Study the drawing (mm; zero at the part's minimum x, y, z) and answer. A direction names the side the tool comes from. Coordinates: 2 decimals unless noted, no trailing zeros. Write each loop counter-clockwise with the first axis right and the second up, starting at its lowest first coordinate (ties: lowest second). Pieces come first, ordered by that corner, then holes. Notation, with made-up numbers: (79, 81.5) -> (125, 81.5) arc R26 ccw to (125, 102.5) -> close; hole circle Ø6 at (-38, 77.25). An arc over 180 degrees is marked (long way). Answer in a Markdown table with one row per item. Add a question column.
Item 1: Given pin 1 Ø1 at (x, y) = (32, 1) entering from +Z; pin 2 Ø0.8 at (y, z) = (1.5, 25.5) entering from -X; pin 3 Ø1 at (x, y) = (10.5, 1) entering from +Z, each flat-ended and moving along its own axis, determine where each tip first touches the part or whether it passes through.
Item 2: For a pull along X with two mould halves and no side action, classify the marked faces 5, 6, 7 and 8 as +X half, -X half, draft (parallel to the pull), parting line (faces both ways), or undercut.
Item 3: Section C-C on z = 31 is taken. Write down the section's boundary in (x, y), then the cut area to 3 significant figures.
Item 4: Section B-B on x = 9.5 is taken. Write down the section's boundary in (y, z), then the cut area to 3 significant figures.
Item 5: Which of the six approach directions +Z, -Z, +X, -X, +Y, -Y give full straight-line access (tool end or side, diameter ignored) to the marked faces 1, 2, 3 and 4?
Item 6: Section A-A on y = 2.6 is taken. Write down the section's boundary in (x, z), then the cut area to 3 significant figures.
Item 7: Straight lines are drawn through the part: line 1 (Z direction, x = 6.5, y = 0.2); line 2 (Z direction, x = 22.5, y = 1.3); line 3 (X direction, y = 0.15, z = 2.5). For each, find the intervals that lie inside material, in ascending order. Write a range as from..to.
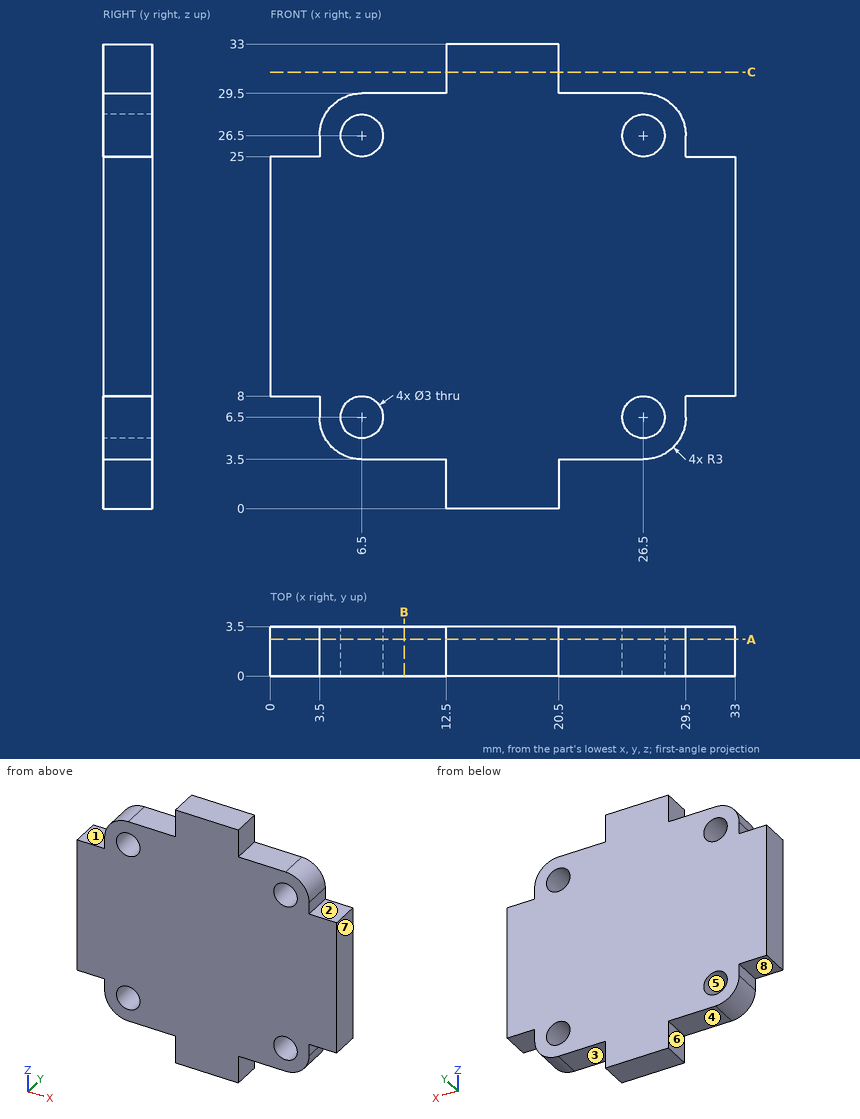
Results below:
| question | item | result |
|---|---|---|
| 1 | pin 1 | stops at z = 25 |
| 1 | pin 2 | stops at x = 3.5 |
| 1 | pin 3 | stops at z = 29.5 |
| 2 | face 5 | undercut |
| 2 | face 6 | -X half |
| 2 | face 7 | +X half |
| 2 | face 8 | draft |
| 3 | outline | (12.5, 0) -> (20.5, 0) -> (20.5, 3.5) -> (12.5, 3.5) -> close |
| 3 | area | 28.0 mm2 |
| 4 | outline | (0, 3.5) -> (3.5, 3.5) -> (3.5, 29.5) -> (0, 29.5) -> close |
| 4 | area | 91.0 mm2 |
| 5 | face 1 | +Z, -X, +Y, -Y |
| 5 | face 2 | +Z, +X, +Y, -Y |
| 5 | face 3 | -Z, +X, +Y, -Y |
| 5 | face 4 | -Z, -X, +Y, -Y |
| 6 | outline | (0, 8) -> (3.5, 8) -> (3.5, 6.5) arc R3 ccw to (6.5, 3.5) -> (12.5, 3.5) -> (12.5, 0) -> (20.5, 0) -> (20.5, 3.5) -> (26.5, 3.5) arc R3 ccw to (29.5, 6.5) -> (29.5, 8) -> (33, 8) -> (33, 25) -> (29.5, 25) -> (29.5, 26.5) arc R3 ccw to (26.5, 29.5) -> (20.5, 29.5) -> (20.5, 33) -> (12.5, 33) -> (12.5, 29.5) -> (6.5, 29.5) arc R3 ccw to (3.5, 26.5) -> (3.5, 25) -> (0, 25) -> close; hole circle Ø3 at (6.5, 6.5); hole circle Ø3 at (6.5, 26.5); hole circle Ø3 at (26.5, 6.5); hole circle Ø3 at (26.5, 26.5) |
| 6 | area | 815 mm2 |
| 7 | line 1 | z = 3.5..5, 8..25, 28..29.5 |
| 7 | line 2 | z = 3.5..29.5 |
| 7 | line 3 | x = 12.5..20.5 |
